Autodesk Inventor part; units mm, degrees
ref_plane "Work Plane_ConnX" through (-32, 0, 0) normal (1, 0, 0) x (0, 1, 0)
ref_plane "Work Plane_ConnY" through (0, 0, 0) normal (0, 1, 0) x (-1, 0, 0)
ref_plane "Work Plane13" through (0, 46, 1.5875) normal (1, 0, 0) x (0, -1, 0)
sketch "Sketch1" plane through (0, 0, 0) normal (0, 0, 1) x (1, 0, 0)
  line L0 (-46, 46) -> (46, 46)
  line L1 (46, 46) -> (46, -46)
  line L2 (46, -46) -> (-46, -46)
  line L3 (-46, -46) -> (-46, 46)
  circle A0 centre (39.5, 39.5) radius 1.5875
  circle A1 centre (-39.5, 39.5) radius 1.5875
  circle A2 centre (-39.5, -39.5) radius 1.5875
  circle A3 centre (39.5, -39.5) radius 1.5875
  line L4 (0, 10.5587) -> (0, 0)
  line L5 (0, 0) -> (12.3531, 0)
  circle A4 centre (-39.5, 39.5) radius 3.175 construction
  line L6 (-38, 44.6281) -> (-38, 37.8613) construction
  dimension "d0" = 92
  dimension "d1" = 92
  dimension "d508" = 3.175
  dimension "d509" = 79
  dimension "d510" = 79
  dimension "d511" = 6.35
  dimension "d515" = 76
extrude "Extrusion1" add sketch "Sketch1" along normal blind 1.5875
ref_plane "Work Plane_ConnX" through (-32, 0, 0) normal (1, 0, 0) x (0, 1, 0)
ref_plane "Work Plane_ConnY" through (0, 0, 0) normal (0, 1, 0) x (-1, 0, 0)
sketch "Sketch9" plane through (0, 0, 1.5875) normal (0, 0, 1) x (1, 0, 0)
  line L0 (46, 46) -> (46, -46)
  line L1 (58.5598, -32) -> (-58.5598, -32)
  circle A0 centre (-2.667, -21.935) radius 0.51
  circle A1 centre (-2.667, -42.065) radius 0.51
  line L2 (0, 26.5598) -> (0, -90.5598) construction
  point P0 (0, 0)
  point P1 (0, -32)
  dimension "d134" = 20.13
  dimension "d136" = 2.667
  dimension "d138" = 1.02
  dimension "d141" = 180
  dimension "d350" = 32
  dimension "d351" = 0
extrude "Holes_Conn_Zminus" cut sketch "Sketch9" against normal through all
sketch "Sketch22" plane through (0, 0, 1.5875) normal (0, 0, 1) x (1, 0, 0)
  line L0 (46, 46) -> (46, -46)
  line L1 (0, -1.0026) -> (0, -62.9974) construction
  line L2 (62.8115, -32) -> (-62.8115, -32)
  circle A0 centre (2.032, -22.7608) radius 0.51
  circle A1 centre (2.032, -41.2392) radius 0.51
  point P0 (46, -35)
  point P1 (46, 35)
  point P2 (0, 0)
  point P3 (0, -32)
  dimension "d282" = 180
  dimension "d283" = 18.4785
  dimension "d284" = 1.02
  dimension "d285" = 2.032
  dimension "d352" = 32
  dimension "d353" = 0
extrude "Holes_Conn_Zplus" cut sketch "Sketch22" against normal through all
chamfer "Chamfer4" distance 8.5 angle 45 4 edges at (-46, 46, 0.7937) (46, 46, 0.7937) (46, -46, 0.7937) (-46, -46, 0.7937)
sketch "Sketch31" plane through (0, 0, 1.5875) normal (0, 0, 1) x (1, 0, 0)
  circle A0 centre (39.5, -39.5) radius 3.175
  circle A1 centre (39.5, 39.5) radius 3.175
  circle A2 centre (-39.5, 39.5) radius 3.175
  circle A3 centre (-39.5, -39.5) radius 3.175
  point P0 (0, 0)
  dimension "d287" = 0
  dimension "d516" = 6.35
sketch "Sketch32" plane through (0, 0, 1.5875) normal (0, 0, 1) x (1, 0, 0)
  line L0 (34, -46) -> (34, -37.2218)
  line L1 (34, -37.2218) -> (37.2218, -34)
  line L2 (37.2218, -34) -> (46, -34)
  line L3 (46, 34) -> (37.2218, 34)
  line L4 (37.2218, 34) -> (34, 37.2218)
  line L5 (34, 37.2218) -> (34, 46)
  line L6 (-34, 46) -> (-34, 37.2218)
  line L7 (-34, 37.2218) -> (-37.2218, 34)
  line L8 (-37.2218, 34) -> (-46, 34)
  line L9 (-34, -46) -> (-34, -37.2218)
  line L10 (-34, -37.2218) -> (-37.2218, -34)
  line L11 (-37.2218, -34) -> (-46, -34)
  point P0 (39.5, -39.5)
  point P1 (0, 0)
  dimension "d287" = 0
  dimension "d519" = 5.5
  dimension "d520" = 5.5
sketch "Sketch34" plane through (0, 0, 1.5875) normal (0, 0, 1) x (1, 0, 0)
  line L0 (37.5, -46) -> (-37.5, -46)
  line L1 (46, 37.5) -> (46, -37.5)
  line L2 (-37.5, 46) -> (37.5, 46)
  line L3 (-46, -37.5) -> (-46, 37.5)
  line L4 (-46, 46) -> (46, 46) construction
  line L5 (46, 46) -> (46, -46) construction
  line L6 (46, -46) -> (-46, -46) construction
  line L7 (-46, -46) -> (-46, 46) construction
  point P0 (0, 0)
decal "Decal4"
sketch "Sketch35" plane through (0, 0, 0) normal (0, 0, -1) x (-1, 0, 0)
  line L0 (46, -37.5) -> (46, 37.5)
  line L1 (37.5, 46) -> (-37.5, 46)
  line L2 (-46, 37.5) -> (-46, -37.5)
  line L3 (-37.5, -46) -> (37.5, -46)
  line L4 (-46, 46) -> (46, 46) construction
  line L5 (46, 46) -> (46, -46) construction
  line L6 (46, -46) -> (-46, -46) construction
  line L7 (-46, -46) -> (-46, 46) construction
  point P0 (0, 0)
decal "Decal5"
sketch "Sketch36" plane through (0, 0, 1.5875) normal (0, 0, 1) x (1, 0, 0)
  line L0 (-37.5, 46) -> (37.5, 46)
  line L1 (37.5, -46) -> (-37.5, -46)
  line L2 (-46, -37.5) -> (-46, 37.5)
  line L3 (46, 37.5) -> (46, -37.5)
  point P0 (0, 0)
  point P1 (0, 46)
  point P2 (0, -46)
  point P3 (-46, 0)
  point P4 (46, 0)
ref_plane "Work Plane13" through (0, 46, 1.5875) normal (1, 0, 0) x (0, -1, 0)
ref_plane "Work Plane14" through (-46, 0, 1.5875) normal (0, 1, 0) x (1, 0, 0)
properties part number "PCB_RT-IHU" material "FR4"
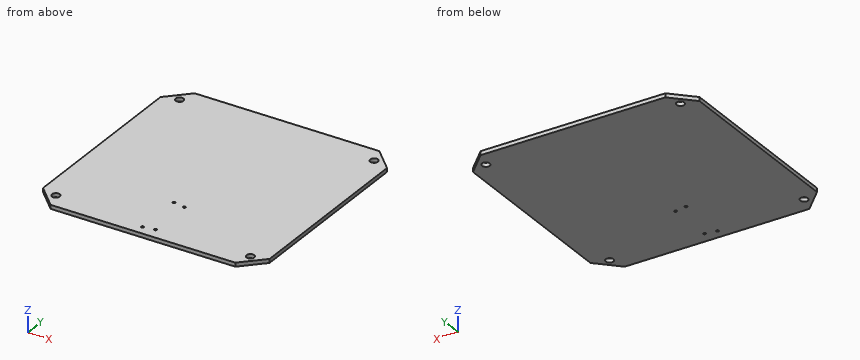
Geometry: final body of the model. Coordinates: model frame, mm. Give positions to 0.01 mm unless a question says otherwise; leave off trailing zeros. Loops run counter-clockwise (first coordinate to the right, second up) from the corner with the lowest first, then second, coordinate; pieces in that order, holes last. Notation, with made-up numbers: (19.5, 17.5) -> (39.5, 17.5) arc R18 cw to (39.5, 31.5) -> close; hole circle Ø1 at (2, 74.5). An arc over 180 degrees is marked (long way). Return JSON: item names as keys, results as strings.
Item 1: Section A-A, the plane x = 39.5. Output: boundary loops of the cut face in (y, z), plus the area to 3 significant figures.
Filled in:
{"outline": "(-44, 0) -> (-41.09, 0) -> (-41.09, 1.59) -> (-44, 1.59) -> close; (-37.91, 0) -> (37.91, 0) -> (37.91, 1.59) -> (-37.91, 1.59) -> close; (41.09, 0) -> (44, 0) -> (44, 1.59) -> (41.09, 1.59) -> close", "area": "130 mm^2"}
Item 2: Pin query (flat end, axial travel): P1, Ø1.3, axis at x = -2.667, y = -21.935, coming from the -Z side. Return the tip coordinate at first contact, or that it passes through.
Filled in:
{"P1": "z = 0"}
Item 3: Line query: line 1 (Y direction, x = 39.5, z = 1.25). Output: solid intervals per line, ascending.
Filled in:
{"line 1": "-44 to -41.09, -37.91 to 37.91, 41.09 to 44"}
Item 4: Section C-C, the plane z = 0.6. Count the separate pieces of the cut face and the enclosed holes in it, plus the area to 3 significant figures.
Filled in:
{"separate pieces": "1", "enclosed holes": "8", "area": "8,280 mm^2"}
